Read the model definition and answer for the solid it produces. Units are mm, in the model's axes. A direction names the side the tool comes from. Give positions to 0.01 mm unless a question says otherwise; leave off trailing zeros. Write each loop counter-clockwise with the first axis right and the second up, starting at its lowest first coordinate (ties: lowest second). Pieces come first, ordered by that corner, then holes. Notation, with made-up numbers: (-36.5, 50.25) - (20.5, 50.25) arc R31 ccw to (20.5, 88.25) - close; hole circle Ø6 at (17.5, -12). An arc over 180 degrees is marked (long way). Answer as a JSON object with one key per item and string values. Group by question number.
```python
from build123d import *

# Parameters (mm, degrees)
SKETCH_R        = 50.5
SKETCH_R_2      = 45.5
PAD_DEPTH       = 60
SKETCH002_R     = 1.5
SKETCH002_R_2   = 10
POCKET_DEPTH    = 8
SKETCH003_R     = 1.5
POCKET001_DEPTH = 8
SKETCH004_R     = 1.5
POCKET002_DEPTH = 5
SKETCH005_R     = 50.5
PAD001_DEPTH    = 2
CHAMFER_SIZE    = 1
CHAMFER001_SIZE = 1


with BuildPart() as part:
    # Sketch → Pad (new body)
    with BuildSketch(Plane.XY):
        Circle(SKETCH_R)
        Circle(SKETCH_R_2, mode=Mode.SUBTRACT)
    extrude(amount=PAD_DEPTH)

    # Sketch002 (on DatumPlane) → Pocket (cut)
    with BuildSketch(Plane(origin=(50.5, 0, 60), x_dir=(0, 1, 0), z_dir=(-1, 0, 0))):
        with Locations((0, 3.8)):
            Circle(SKETCH002_R)
        with Locations((0, 18)):
            Circle(SKETCH002_R_2)
        with BuildLine():
            Line((0, 47.6), (0.0005, 47.6))
            ThreePointArc((0.0005, 47.6), (1.060807, 48.039193), (1.5, 49.0995))
            Line((1.5, 49.0995), (1.5, 52.1005))
            ThreePointArc((1.5, 52.1005), (1.060807, 53.160807), (0.0005, 53.6))
            Line((0.0005, 53.6), (0, 53.6))
            ThreePointArc((0, 53.6), (-1.06066, 53.16066), (-1.5, 52.1))
            Line((-1.5, 52.1), (-1.5, 49.1))
            ThreePointArc((-1.5, 49.1), (-1.06066, 48.03934), (0, 47.6))
        make_face()
    extrude(amount=POCKET_DEPTH, mode=Mode.SUBTRACT)

    # Sketch003 (on DatumPlane) → Pocket001 (cut)
    with BuildSketch(Plane(origin=(0, 50.5, 60), x_dir=(0, 0, -1), z_dir=(0, 1, 0))):
        with Locations((3.8, 0)):
            Circle(SKETCH003_R)
        with Locations((24.8, 0)):
            Circle(SKETCH003_R)
    extrude(amount=-POCKET001_DEPTH, mode=Mode.SUBTRACT)

    # Sketch004 (on DatumPlane) → Pocket002 (cut)
    with BuildSketch(Plane(origin=(0, -50.5, 60), x_dir=(0, 0, 1), z_dir=(0, -1, 0))):
        with Locations((-3.8, 0)):
            Circle(SKETCH004_R)
        with Locations((-24.8, 0)):
            Circle(SKETCH004_R)
        with BuildLine():
            Line((-52.1, -1.5), (-49.095, -1.5))
            ThreePointArc((-49.095, -1.5), (-48.037875, -1.062125), (-47.6, -0.005))
            Line((-47.6, -0.005), (-47.6, 0))
            ThreePointArc((-47.6, 0), (-48.03934, 1.06066), (-49.1, 1.5))
            Line((-49.1, 1.5), (-52.105, 1.5))
            ThreePointArc((-52.105, 1.5), (-53.162125, 1.062125), (-53.6, 0.005))
            Line((-53.6, 0.005), (-53.6, 0))
            ThreePointArc((-53.6, 0), (-53.16066, -1.06066), (-52.1, -1.5))
        make_face()
    extrude(amount=-POCKET002_DEPTH, mode=Mode.SUBTRACT)

    # Sketch005 (on Face8 of Pocket002) → Pad001 (join)
    with BuildSketch(Plane.XY.offset(60)):
        Circle(SKETCH005_R)
    extrude(amount=PAD001_DEPTH)

    # Chamfer
    chamfer_edges = [part.edges().sort_by_distance(p)[0] for p in [
        (-50.5, 0, 62),
    ]]
    chamfer(chamfer_edges, length=CHAMFER_SIZE)

    # Chamfer001
    chamfer001_edges = [part.edges().sort_by_distance(p)[0] for p in [
        (-45.5, 0, 0),
    ]]
    chamfer(chamfer001_edges, length=CHAMFER001_SIZE)


solid = part.part
```
1) Find the intervals of material crossed by line 1 (Z direction, x = 0, y = 48.45); line 2 (Z direction, x = 46.8, y = 0); line 3 (Y direction, x = 38.5, z = 18.5), in increasing order. Write a range as [from, to].
2) Flat-ended cylindrical pins translate along their axes: pin 1 Ø1.7 at (x, z) = (1, 56.5) entering from -Y; pin 2 Ø0.5 at (x, z) = (0.5, 10) entering from -Y; pin 3 Ø10 at (x, z) = (11, 15) entering from +Y. Find the tip coordinate at first contact, or state that the pin passes through.
3) Which of the six approach directions +Z, -Z, +X, -X, +Y, -Y give full straight-line access (tool end or side, diameter ignored) to faces 1 (the flat face through (-1.5, -48, 9)), 2 (the cylindrical face through (-36.107, -27.686, 30.087)), 3 (the cylindrical face through (48.023, -0.325, 57.664))?
4) Find section C-C, the plane z = 42. Write down the section's boundary in (x, y).
5) For a pull along Y with two mould halves and no side action, classify faces 4 (the cylindrical face through (0.9, -48, 55)), 5 (the flat face through (48, -1.5, 9)), 6 (the cylindrical face through (-10.95, -49.3, 30.07)) as released by +Y, released by -Y, zero draft, split by the parting line, or undercut.
Values follow:
{
 "1": {"line 1": "z = [0, 33.7], [36.7, 54.7], [57.7, 62]", "line 2": "z = [0, 6.4], [12.4, 32], [52, 54.7], [57.7, 62]", "line 3": "y = [-32.68, -24.25], [24.25, 32.68]"},
 "2": {"pin 1": "stops at y = -50.49", "pin 2": "stops at y = -45.5", "pin 3": "stops at y = 50.14"},
 "3": {"face 1": "-Y", "face 2": "-Z", "face 3": "+X"},
 "4": {"outline": "(44.39, -10) arc R45.5 cw (long way) to (44.39, 10) - (49.5, 10) arc R50.5 ccw (long way) to (49.5, -10) - close"},
 "5": {"face 4": "zero draft", "face 5": "undercut", "face 6": "split by the parting line"}
}
